from build123d import *

# Parameters (mm, degrees)
BASEHEAD_DEPTH = 6.58
SKETCH3_R      = 5
BASEBODY_DEPTH = 40
CHAMFER1_SIZE  = 0.812


with BuildPart() as part:
    # Sketch-BaseHead → BaseHead (new body)
    with BuildSketch(Plane(origin=(0, 0, 0), x_dir=(0, 0, -1), z_dir=(1, 0, 0))):
        Polygon((9.081719734, 0), (4.540859867, 7.865), (-4.540859867, 7.865), (-9.081719734, 0), (-4.540859867, -7.865), (4.540859867, -7.865), align=None)
    extrude(amount=BASEHEAD_DEPTH)

    # Sketch4 → HeadChamfer (revolve, cut)
    with BuildSketch(Plane(origin=(-0.264637255, 0, 5.916896391), x_dir=(0, 0, -1), z_dir=(0, 1, 0))):
        Polygon((14.998616125, -0.264637255), (13.781896391, -0.264637255), (14.998616125, -0.707487022), align=None)
    revolve(axis=Axis((-4.001564945, 0, 0), (1, 0, 0)), mode=Mode.SUBTRACT)

    # Sketch1 → Revolve1 (revolve)
    with BuildSketch(Plane.XY):
        Polygon((6.58, 0), (7.08, 0), (7.08, -7.315), (6.58, -7.865), align=None)
    revolve(axis=Axis((-4.001564945, 0, 0), (1, 0, 0)))

    # Sketch3 → BaseBody (add)
    with BuildSketch(Plane(origin=(7.08, 0, 0), x_dir=(0, 0, -1), z_dir=(1, 0, 0))):
        Circle(SKETCH3_R)
    extrude(amount=BASEBODY_DEPTH)

    # Chamfer1
    chamfer1_edges = [part.edges().sort_by_distance(p)[0] for p in [
        (47.08, 0, 5),
    ]]
    chamfer(chamfer1_edges, length=CHAMFER1_SIZE)


solid = part.part
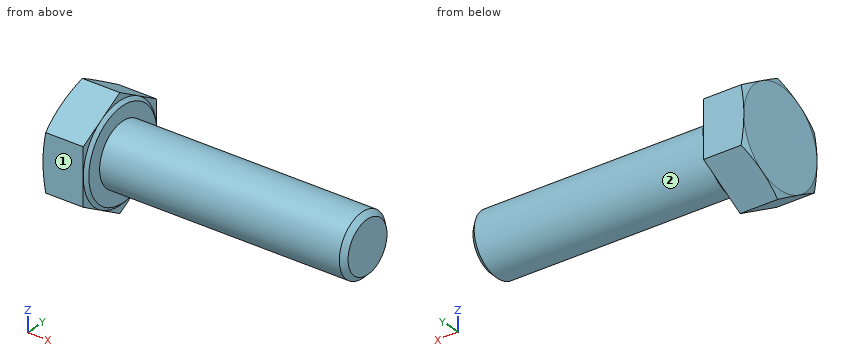
Work out the finished part from the listing and answer in its coordinate system (mm). Face numbers are marked on the shaded views. A direction names the side the tool comes from. Round coordinates to 2 decimals unless told otherwise and drop trailing zeros. Order: outer loops, then holes, each group sorted by start corner. A loop starts at its lowest first (then second) coordinate and runs counter-clockwise, first axis right, second up. Notation, with made-up numbers: M -0.5,-33 L 41.5,-33 A18 cw 41.5,-23 Z; hole C -5,42.5 d3. An arc over 180 degrees is marked long. Put each result on its own line as item: value. Start each with the question number.
Q1. Section A-A, the plane x = 5.5 is taken. Write down the section's boundary in (y, z) (3 decimals), and give its area (3 significant figures).
Q2. Flat-ended cylindrical pins translate along their axes: pin 1 (4.5 mm diameter, centred on y = -6, z = -3.5, fed in from +X); pin 2 (1.5 mm diameter, centred on x = 24.5, z = 3, fed in from +Y); pin 3 (1.5 mm diameter, centred on y = -0.5, z = -5.5, fed in from +X). Find the tip coordinate at first contact, or state that the pin passes through.
Q3. A tool of negligible diameter and unlimited length cuts with its end or side. For the marked faces 1 and 2, from which of +Z, -Z, +X, -X, +Y, -Y can it reach the whole face along a straight path? Write none if from no direction.
Q4. Section B-B, the plane x = 39.5 is taken. Write down the section's boundary in (y, z), and give its area (3 significant figures).
Q5. Straight lines are drawn through the part: L1, parallel to Z at x = 39.5, y = -0.25; L2, parallel to X at y = -4.5, z = -2.25; L3, parallel to Y at x = 7.5, z = 0. For each, find the intervals that lie inside material, in ascending order. Write a range as [from, to].
Findings below:
1. outline: M -7.865,-4.541 L 0,-9.082 L 7.865,-4.541 L 7.865,4.541 L 0,9.082 L -7.865,4.541 Z
1. area: 214 mm^2
2. pin 1: stops at x = 46.57
2. pin 2: stops at y = 4.47
2. pin 3: stops at x = 46.5
3. face 1: +Z, -Z, +X, -X, -Y
3. face 2: +X
4. outline: C 0,0 d10
4. area: 78.5 mm^2
5. L1: z = [-4.99, 4.99]
5. L2: x = [0, 7.08]
5. L3: y = [-5, 5]
